Part model, mm, in its own coordinate system. A direction names the side the tool comes from. Give positions to 0.01 mm unless a question says otherwise; leave off trailing zeros. Write each loop counter-clockwise with the first axis right and the second up, starting at its lowest first coordinate (ties: lowest second). Pieces come first, ordered by that corner, then holes. Notation, with made-up numbers: M 73,4.5 L 77,4.5 A24 ccw 77,26.5 Z; hole C 11.25,39 d10. An arc over 180 degrees is marked long. Use a Markdown table: item, result.
```python
from build123d import *

# Parameters (mm, degrees)
F0_R     = 1.5875
F1_DEPTH = 12.7


with BuildPart() as f1:
    # F0 (on Top) → F1 (new body)
    with BuildSketch(Plane.XY):
        with BuildLine():
            ThreePointArc((3.011577, -1.0055), (3.133878, -0.509347), (3.175, 0))
            ThreePointArc((3.175, 0), (3.133878, 0.509347), (3.011577, 1.0055))
            ThreePointArc((3.011577, 1.0055), (2.749631, 1.5875), (2.376577, 2.105352))
            ThreePointArc((2.376577, 2.105352), (1.5875, 2.749631), (0.635, 3.110852))
            ThreePointArc((0.635, 3.110852), (0, 3.175), (-0.635, 3.110852))
            ThreePointArc((-0.635, 3.110852), (-1.5875, 2.749631), (-2.376577, 2.105352))
            ThreePointArc((-2.376577, 2.105352), (-2.749631, 1.5875), (-3.011577, 1.0055))
            ThreePointArc((-3.011577, 1.0055), (-3.175, 0), (-3.011577, -1.0055))
            ThreePointArc((-3.011577, -1.0055), (-2.749631, -1.5875), (-2.376577, -2.105352))
            ThreePointArc((-2.376577, -2.105352), (-1.5875, -2.749631), (-0.635, -3.110852))
            ThreePointArc((-0.635, -3.110852), (0, -3.175), (0.635, -3.110852))
            ThreePointArc((0.635, -3.110852), (1.5875, -2.749631), (2.376577, -2.105352))
            ThreePointArc((2.376577, -2.105352), (2.749631, -1.5875), (3.011577, -1.0055))
        make_face()
        Circle(F0_R, mode=Mode.SUBTRACT)
        with BuildLine():
            ThreePointArc((2.376577, 2.105352), (2.749631, 1.5875), (3.011577, 1.0055))
            Line((3.011577, 1.0055), (8.621946, 4.244648))
            ThreePointArc((8.621946, 4.244648), (8.248892, 4.7625), (7.986946, 5.3445))
            Line((7.986946, 5.3445), (2.376577, 2.105352))
        make_face()
        with BuildLine():
            Line((8.621946, -4.244648), (3.011577, -1.0055))
            ThreePointArc((3.011577, -1.0055), (2.749631, -1.5875), (2.376577, -2.105352))
            Line((2.376577, -2.105352), (7.986946, -5.3445))
            ThreePointArc((7.986946, -5.3445), (8.248892, -4.7625), (8.621946, -4.244648))
        make_face()
        with BuildLine():
            ThreePointArc((7.986946, 5.3445), (8.248892, 4.7625), (8.621946, 4.244648))
            ThreePointArc((8.621946, 4.244648), (12.124354, 3.381309), (14.173523, 6.35))
            ThreePointArc((14.173523, 6.35), (10.489176, 9.483878), (7.986946, 5.3445))
        make_face()
        with Locations((10.998523, 6.35)):
            Circle(F0_R, mode=Mode.SUBTRACT)
        with BuildLine():
            ThreePointArc((14.173523, -6.35), (12.124354, -3.381309), (8.621946, -4.244648))
            ThreePointArc((8.621946, -4.244648), (8.248892, -4.7625), (7.986946, -5.3445))
            ThreePointArc((7.986946, -5.3445), (10.489176, -9.483878), (14.173523, -6.35))
        make_face()
        with Locations((10.998523, -6.35)):
            Circle(F0_R, mode=Mode.SUBTRACT)
        with BuildLine():
            ThreePointArc((-0.635, 3.110852), (0, 3.175), (0.635, 3.110852))
            Line((0.635, 3.110852), (0.635, 9.589148))
            ThreePointArc((0.635, 9.589148), (0, 9.525), (-0.635, 9.589148))
            Line((-0.635, 9.589148), (-0.635, 3.110852))
        make_face()
        with BuildLine():
            Line((0.635, -9.589148), (0.635, -3.110852))
            ThreePointArc((0.635, -3.110852), (0, -3.175), (-0.635, -3.110852))
            Line((-0.635, -3.110852), (-0.635, -9.589148))
            ThreePointArc((-0.635, -9.589148), (0, -9.525), (0.635, -9.589148))
        make_face()
        with BuildLine():
            ThreePointArc((-0.635, 9.589148), (0, 9.525), (0.635, 9.589148))
            ThreePointArc((0.635, 9.589148), (2.459344, 10.691954), (3.175, 12.7))
            ThreePointArc((3.175, 12.7), (-2.008046, 15.159344), (-0.635, 9.589148))
        make_face()
        with Locations((0, 12.7)):
            Circle(F0_R, mode=Mode.SUBTRACT)
        with BuildLine():
            ThreePointArc((3.175, -12.7), (2.459344, -10.691954), (0.635, -9.589148))
            ThreePointArc((0.635, -9.589148), (0, -9.525), (-0.635, -9.589148))
            ThreePointArc((-0.635, -9.589148), (-2.008046, -15.159344), (3.175, -12.7))
        make_face()
        with Locations((0, -12.7)):
            Circle(F0_R, mode=Mode.SUBTRACT)
        with BuildLine():
            ThreePointArc((-3.011577, 1.0055), (-2.749631, 1.5875), (-2.376577, 2.105352))
            Line((-2.376577, 2.105352), (-7.986946, 5.3445))
            ThreePointArc((-7.986946, 5.3445), (-8.248892, 4.7625), (-8.621946, 4.244648))
            Line((-8.621946, 4.244648), (-3.011577, 1.0055))
        make_face()
        with BuildLine():
            Line((-7.986946, -5.3445), (-2.376577, -2.105352))
            ThreePointArc((-2.376577, -2.105352), (-2.749631, -1.5875), (-3.011577, -1.0055))
            Line((-3.011577, -1.0055), (-8.621946, -4.244648))
            ThreePointArc((-8.621946, -4.244648), (-8.248892, -4.7625), (-7.986946, -5.3445))
        make_face()
        with BuildLine():
            ThreePointArc((-8.621946, 4.244648), (-8.248892, 4.7625), (-7.986946, 5.3445))
            ThreePointArc((-7.986946, 5.3445), (-7.864645, 5.840653), (-7.823523, 6.35))
            ThreePointArc((-7.823523, 6.35), (-13.967214, 7.475832), (-8.621946, 4.244648))
        make_face()
        with Locations((-10.998523, 6.35)):
            Circle(F0_R, mode=Mode.SUBTRACT)
        with BuildLine():
            ThreePointArc((-7.823523, -6.35), (-7.864645, -5.840653), (-7.986946, -5.3445))
            ThreePointArc((-7.986946, -5.3445), (-8.248892, -4.7625), (-8.621946, -4.244648))
            ThreePointArc((-8.621946, -4.244648), (-13.967214, -7.475832), (-7.823523, -6.35))
        make_face()
        with Locations((-10.998523, -6.35)):
            Circle(F0_R, mode=Mode.SUBTRACT)
    extrude(amount=F1_DEPTH)


solid = f1.part
```
1. Cut at D-D, the plane y = -9. Give the cut face in (x, z) (3 decimals).
Findings below:
| item | result |
|---|---|
| outline | M -12.747,0 L -9.25,0 L -9.25,12.7 L -12.747,12.7 Z; M -0.635,0 L 0.635,0 L 0.635,12.7 L -0.635,12.7 Z; M 9.25,0 L 12.747,0 L 12.747,12.7 L 9.25,12.7 Z |
2. Cut at C-C, the plane z = 5. State how many separate pieces and enclosed holes the cut face has, then the cut area to 3 significant figures.
Findings below:
| item | result |
|---|---|
| separate pieces | 1 |
| enclosed holes | 7 |
| area | 215 mm2 |
3. Cut at A-A, the plane x = 0. Give the cut face in (y, z) (1 decimal).
Findings below:
| item | result |
|---|---|
| outline | M -15.9,0 L -14.3,0 L -14.3,12.7 L -15.9,12.7 Z; M -11.1,0 L -1.6,0 L -1.6,12.7 L -11.1,12.7 Z; M 1.6,0 L 11.1,0 L 11.1,12.7 L 1.6,12.7 Z; M 14.3,0 L 15.9,0 L 15.9,12.7 L 14.3,12.7 Z |
4. Drop flat-ended pins along their axis: P1, Ø1, axis at y = 1, z = 3, coming from the +X side; P2, Ø2.5, axis at x = 11, y = -6.35, coming from the -Z side; P3, Ø5, axis at y = -11.5, z = 2.5, coming from the +X side; P4, Ø4, axis at y = -0.5, z = 7, coming from the -X side. Give the stop position or say it passes through.
Findings below:
| item | result |
|---|---|
| P1 | x = 3.87 |
| P2 | through |
| P3 | x = 12.75 |
| P4 | x = -5.6 |
5. Cut at B-B, the plane y = 7.5. Give the cut face in (x, z) (3 decimals).
Findings below:
| item | result |
|---|---|
| outline | M -13.958,0 L -12.093,0 L -12.093,12.7 L -13.958,12.7 Z; M -9.904,0 L -8.039,0 L -8.039,12.7 L -9.904,12.7 Z; M -0.635,0 L 0.635,0 L 0.635,12.7 L -0.635,12.7 Z; M 8.039,0 L 9.904,0 L 9.904,12.7 L 8.039,12.7 Z; M 12.093,0 L 13.958,0 L 13.958,12.7 L 12.093,12.7 Z |
6. Drill centre lines: L1, parallel to Y at x = 0, z = 9 (1 decimal); L2, parallel to Y at x = -10, z = 4; L3, parallel to X at y = -3.5, z = 8.75 (3 decimals). Where is each one in solid material? Low to high.
Findings below:
| item | result |
|---|---|
| L1 | -15.9 to -14.3, -11.1 to -1.6, 1.6 to 11.1, 14.3 to 15.9 |
| L2 | -9.36 to -7.58, -5.12 to -3.34, 3.34 to 5.12, 7.58 to 9.36 |
| L3 | -12.398 to -9.599, -7.332 to -4.792, -0.635 to 0.635, 4.792 to 7.332, 9.599 to 12.398 |
7. Tool access for faces 1 (the cylindrical face through (1.575, -2.757, 6.261)), 2 (the flat face through (2, 0, 12.7)): list every direction of +Z, -Z, +X, -X, +Y, -Y with a clear straight run to the whole face (end or side of a thin tool).
Findings below:
| item | result |
|---|---|
| face 1 | +Z, -Z |
| face 2 | +Z, +X, -X, +Y, -Y |
8. Two-plate mould, pull along X, no slides. Class faces 3 (the cylindrical face through (-3.175, 0.014, 6.261)), 4 (the flat face through (-5.777, -2.602, 6.261)), 5 (the flat face through (2, 0, 0)): released by +X, released by -X, zero draft, split by the parting line, or undercut.
Findings below:
| item | result |
|---|---|
| face 3 | released by -X |
| face 4 | undercut |
| face 5 | zero draft |
